from build123d import *

# Parameters (mm, degrees)
F1_DEPTH     = 25.4
F2_R         = 12.7
F3_R         = 12.69999
F4_R         = 12.7
F5_R         = 12.69999
F6_R         = 6.35
F7_DEPTH     = 25.4
F8_W         = 31.75
F8_H         = 12.7
F9_DEPTH     = 25.4
F10_R        = 7.62
F11_T1_DEPTH = 12.7
F12_R        = 7.62
F13_T1_DEPTH = 12.7


# Not quite as in the source:
# - a fillet or chamfer that OpenCascade refuses, or shapes differently, is made with other operations: its cross-section is extruded or revolved along the edge and cut away or added
# - a fillet or chamfer is up to 0.001 mm smaller than in the source, because OpenCascade refuses the exact size


with BuildPart() as f1:
    # F0 (on Front) → F1 (new body)
    with BuildSketch(Plane.XZ):
        Polygon((0, 38.1), (0, 0), (69.85, 0), (69.85, 12.7), (25.4, 12.7), (25.4, 38.1), align=None)
    extrude(amount=F1_DEPTH)

    # F2
    f2_edges = [f1.edges().sort_by_distance(p)[0] for p in [
        (69.85, -25.4, 6.35),
    ]]
    fillet(f2_edges, radius=F2_R)

    # F3 (radius 12.7 in the source; OpenCascade refuses exactly that, so slightly less here)
    f3_edges = [f1.edges().sort_by_distance(p)[0] for p in [
        (69.85, 0, 6.35),
    ]]
    fillet(f3_edges, radius=F3_R)

    # F4
    f4_edges = [f1.edges().sort_by_distance(p)[0] for p in [
        (25.4, -12.7, 38.1),
    ]]
    fillet(f4_edges, radius=F4_R)

    # F5 (radius 12.7 in the source; OpenCascade refuses exactly that, so slightly less here)
    f5_edges = [f1.edges().sort_by_distance(p)[0] for p in [
        (0, -12.7, 38.1),
    ]]
    fillet(f5_edges, radius=F5_R)

    # F6 (on face) → F7 (cut)
    with BuildSketch(Plane.XZ.offset(25.4)):
        with Locations((12.7, 25.4)):
            Circle(F6_R)
    extrude(amount=-F7_DEPTH, mode=Mode.SUBTRACT)

    # F8 (on face) → F9 (cut)
    with BuildSketch(Plane.XY.offset(12.7)):
        with Locations((46.4384327233, -12.3384663999)):
            Rectangle(F8_W, F8_H)
    extrude(amount=-F9_DEPTH, mode=Mode.SUBTRACT)

    # F10
    f10_edges = [f1.edges().sort_by_distance(p)[0] for p in [
        (30.563433, -5.988466, 6.35),
    ]]
    fillet(f10_edges, radius=F10_R)

    # F11: fillet of radius 7.62 on 1 edges, made by hand

    # F11_s2 → F11_t1 (join)
    with BuildSketch(Plane.XY):
        with BuildLine():
            ThreePointArc((30.5634327233, -13.6084663999), (33.3482285689, -17.2901703466), (37.7476376201, -18.6884663999))
            Line((37.7476376201, -18.6884663999), (30.5634327233, -18.6884663999))
            Line((30.5634327233, -18.6884663999), (30.5634327233, -13.6084663999))
        make_face()
    extrude(amount=F11_T1_DEPTH)

    # F12
    f12_edges = [f1.edges().sort_by_distance(p)[0] for p in [
        (62.313433, -5.988466, 6.35),
    ]]
    fillet(f12_edges, radius=F12_R)

    # F13: fillet of radius 7.62 on 1 edges, made by hand

    # F13_s2 → F13_t1 (join)
    with BuildSketch(Plane.XY):
        with BuildLine():
            ThreePointArc((62.3134327233, -13.6084663999), (59.5286368777, -17.2901703466), (55.1292278264, -18.6884663999))
            Line((55.1292278264, -18.6884663999), (62.3134327233, -18.6884663999))
            Line((62.3134327233, -18.6884663999), (62.3134327233, -13.6084663999))
        make_face()
    extrude(amount=F13_T1_DEPTH)


solid = f1.part
The model under review builds one solid part; all positions refer to its coordinate system, in mm. A direction names the side the tool comes from. Give positions to 0.01 mm unless a question says otherwise; leave off trailing zeros. Order: outer loops, then holes, each group sorted by start corner. A loop starts at its lowest first (then second) coordinate and runs counter-clockwise, first axis right, second up. Notation, with made-up numbers: M 31,-3 L 66,-3 A23 cw 66,20 Z; hole C 69.5,-28 d3. An arc over 180 degrees is marked long. Answer in a Markdown table with one row per item. Add a question column.
1. To check wall thickness, follow line 1 along Y through (x, z) = (50.5, 6); line 2 along Z through (x, y) = (39, -22.5); line 3 along X through (y, z) = (-12.5, 5). State the ranges of each line that lie inside material, in increasing order.
2. Mouldability with a two-part tool opening along X and no side actions: class faces 1 (the flat face through (47, -4, 12.7)), 2 (the flat face through (0, -13, 13)), 3 (the flat face through (25.4, -13, 19)), 4 (the cylindrical face through (33.29, -17.25, 6.26)) as released by +X, released by -X, zero draft, split by the parting line, or undercut.
3. Add section A-A on y = -16. Count the separate pieces of the cut face and the enclosed holes in it, plus the area to 3 significant figures.
4. Add section C-C on x = 18. State the section outline as (y, z) points, plus the area to 3 significant figures.
5. For pin 1 Ø7.5 at (x, y) = (48, -14.5) entering from +Z; pin 2 Ø12 at (x, y) = (30, -20) entering from +Z; pin 3 Ø4 at (y, z) = (-6.5, 16) entering from +X, all flat-tipped, find the tip position at first contact; note any pin that passes through.
6. Machinability: for faces 5 (the flat face through (27, -13, 0)), 6 (the cylindrical face through (60.02, -8.16, 6.26)), which of the approach directions +Z, -Z, +X, -X, +Y, -Y give a long, thin tool a straight path to every point of the face, cutting with its end or side? Answer none if there is none.
The answers:
| question | item | result |
|---|---|---|
| 1 | line 1 | -25.4 to -18.69, -5.99 to 0 |
| 1 | line 2 | 0 to 12.7 |
| 1 | line 3 | 0 to 30.64, 62.23 to 69.85 |
| 2 | face 1 | zero draft |
| 2 | face 2 | released by -X |
| 2 | face 3 | released by +X |
| 2 | face 4 | undercut |
| 3 | separate pieces | 2 |
| 3 | enclosed holes | 1 |
| 3 | area | 963 mm2 |
| 4 | outline | M -25.4,0 L 0,0 L 0,21.9 L -25.4,21.9 Z; M -25.4,28.9 L 0,28.9 L 0,36.94 L -25.4,36.94 Z |
| 4 | area | 761 mm2 |
| 5 | pin 1 | through |
| 5 | pin 2 | z = 31.2 |
| 5 | pin 3 | x = 25.4 |
| 6 | face 5 | -Z, +X, -X, +Y, -Y |
| 6 | face 6 | +Z, -Z |
